from build123d import *
from build123d.topology import SkipClean

# Parameters (mm, degrees)
BOSS_EXTRUDE1_DEPTH     = 12
CUT_EXTRUDE1_DEPTH      = 22.914607001
CUT_EXTRUDE1_DEPTH_BACK = 22.914607001
SKETCH4_R               = 3
SKETCH4_R_2             = 1.5
BOSS_EXTRUDE2_DEPTH     = 8
SKETCH5_R               = 3
SKETCH5_R_2             = 1.5
CUT_EXTRUDE2_DEPTH      = 2.5
FILLET1_R               = 1
FILLET2_R               = 1
CUT_EXTRUDE3_DEPTH      = 22.914607001
CUT_EXTRUDE3_DEPTH_BACK = 22.914607001
SKETCH6_W               = 12
SKETCH6_H               = 6.5
CUT_EXTRUDE4_DEPTH      = 5
BOSS_EXTRUDE3_REACH     = 24.623
SKETCH8_R               = 1.5
SKETCH9_W               = 2
SKETCH9_H               = 33.212886517
CUT_EXTRUDE5_DEPTH      = 1


with BuildPart() as part:
    # Sketch1 → Boss-Extrude1 (new body)
    with BuildSketch(Plane.XY):
        with BuildLine():
            Line((-8, -10), (8, -10))
            Line((8, -10), (6.5, 10))
            ThreePointArc((6.5, 10), (0, 16.5), (-6.5, 10))
            Line((-6.5, 10), (-8, -10))
        make_face()
    extrude(amount=BOSS_EXTRUDE1_DEPTH)

    # Sketch3 → Cut-Extrude1 (cut, two sides: drawn at the far end of the back side and taken through both)
    with BuildSketch(Plane(origin=(0, 0, 0), x_dir=(0, 0, -1), z_dir=(1, 0, 0)).offset(-CUT_EXTRUDE1_DEPTH_BACK)):
        Polygon((-4, -10), (-12, -3.386045056), (-12, -10), align=None)
    extrude(amount=CUT_EXTRUDE1_DEPTH + CUT_EXTRUDE1_DEPTH_BACK, mode=Mode.SUBTRACT)

    # Sketch4 → Boss-Extrude2 (add, symmetric)
    with BuildSketch(Plane(origin=(0, 0, 0), x_dir=(0, 0, -1), z_dir=(1, 0, 0))):
        with Locations((-6, -11.1)):
            Circle(SKETCH4_R)
        with Locations((-6, -11.1)):
            Circle(SKETCH4_R_2, mode=Mode.SUBTRACT)
    extrude(amount=BOSS_EXTRUDE2_DEPTH, both=True)

    # Sketch5 → Cut-Extrude2 (cut, symmetric)
    with SkipClean():  # the faces are left unmerged after this step: merging them gives an invalid solid
        with BuildSketch(Plane(origin=(0, 0, 0), x_dir=(0, 0, -1), z_dir=(1, 0, 0))):
            with Locations((-6, -11.1)):
                Circle(SKETCH5_R)
            with Locations((-6, -11.1)):
                Circle(SKETCH5_R_2, mode=Mode.SUBTRACT)
        extrude(amount=CUT_EXTRUDE2_DEPTH, both=True, mode=Mode.SUBTRACT)

    # Fillet1
    fillet1_edges = [part.edges().sort_by_distance(p)[0] for p in [
        (5.179248458, -8.113292219, 6.282093298),
        (-5.179248458, -8.113292219, 6.282093298),
    ]]
    fillet(fillet1_edges, radius=FILLET1_R)

    # Fillet2
    # the kernel refuses this fillet: 1 mm, written as the material it adds along each edge
    with BuildSketch(Plane(origin=(-8, -10, 3.208942853), x_dir=(0, 0, -1), z_dir=(1, 0, 0)), Plane(origin=(2.5, -10, 3.208942853), x_dir=(0, 0, -1), z_dir=(1, 0, 0))) as fillet2_piece_1:
        with BuildLine():
            CenterArc((1.207692657, -1), FILLET2_R, 90, 91.432543738)
            ThreePointArc((0.208005206, -1.025), (0.149015506, -0.503365446), (0, 0))
            Line((0, 0), (1.207692657, 0))
        make_face()
    extrude(amount=5.5)

    # Sketch6 → Cut-Extrude3 (cut, two sides: drawn at the far end of the back side and taken through both)
    with BuildSketch(Plane(origin=(0, 0, 0), x_dir=(0, 0, -1), z_dir=(1, 0, 0)).offset(-CUT_EXTRUDE3_DEPTH_BACK)):
        with Locations((-6, 13.25)):
            Rectangle(SKETCH6_W, SKETCH6_H)
    extrude(amount=CUT_EXTRUDE3_DEPTH + CUT_EXTRUDE3_DEPTH_BACK, mode=Mode.SUBTRACT)

    # Sketch7 → Cut-Extrude4 (cut)
    with BuildSketch(Plane(origin=(0, -7.904323178, 6.53485467), x_dir=(1, 0, 0), z_dir=(0, -0.770712909441233, 0.6371825572162423))):
        Polygon((-5, 5.891026066), (0, 5.891026066), (5, 5.891026066), (5, 1.891026066), (-5, 1.891026066), align=None)
    extrude(amount=-CUT_EXTRUDE4_DEPTH, mode=Mode.SUBTRACT)

    # Sketch8 → Boss-Extrude3 (add, up to next)
    with BuildSketch(Plane(origin=(-5, 0, 0), x_dir=(0, 0, -1), z_dir=(1, 0, 0)), mode=Mode.PRIVATE) as boss_extrude3_sk1:
        with Locations(Location((-7.940762297, -3.498246966, 0), (0, 0, 180))):
            Circle(SKETCH8_R)
    boss_extrude3_tool1 = extrude(boss_extrude3_sk1.sketch, amount=BOSS_EXTRUDE3_REACH, mode=Mode.PRIVATE) - part.part
    add(boss_extrude3_tool1.solids().sort_by_distance((-5, -3.498247, 7.940762))[0])

    # Sketch9 → Cut-Extrude5 (cut, symmetric)
    with BuildSketch(Plane(origin=(0, 0, 0), x_dir=(0, 0, -1), z_dir=(1, 0, 0))):
        with Locations((-1.32, 6.606443259)):
            Rectangle(SKETCH9_W, SKETCH9_H)
    extrude(amount=CUT_EXTRUDE5_DEPTH, both=True, mode=Mode.SUBTRACT)


solid = part.part
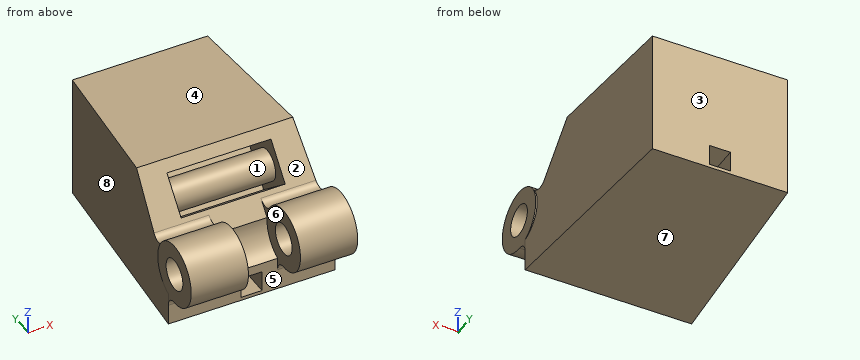
Input: part model. Units: mm. Frame: model coordinates. Face numbers are marked on the shaded views. A direction names the side the tool comes from. Give positions to 0.01 mm unless a question says otherwise; leave off trailing zeros. Order: outer loops, then holes, each group sorted by start corner. A loop starts at its lowest first (then second) coordinate and runs counter-clockwise, first axis right, second up. Notation, with made-up numbers: (65, 54.25) - (119, 54.25) arc R30 cw to (119, 89.25) - close; hole circle Ø5 at (53, -23). An arc over 180 degrees is marked (long way). Answer as a JSON object with one key per item and string values. Group by question number.
Q1. Mould query, pull axis X, two halves, no side actions, for the marked faces 6, 7 and 8. Classes: pulls with the +X half, pulls with the -X half, needs draft (parallel to the pull), parting line crosses it, or undercut.
Q2. Cut plane B-B, the plane z = 8.25. Output: boundary loops of the cut face in (x, y), then the cut area to 3 significant figures.
Q3. Line query: probe 1 along Z at (x, y) = (-3.25, -3); probe 2 along X at (y, z) = (-8.75, 5.5); probe 3 along Y at (x, z) = (6.35, 6). Output: solid intervals per line, ascending.
Q4. Cut plane A-A, the plane x = 4.25. Output: boundary loops of the cut face in (y, z) (3 decimals), then the cut area to 3 significant figures.
Q5. Cut plane C-C, the plane x = -1.75. Output: boundary loops of the cut face in (y, z), then the cut area to 3 significant figures.
Q6. Set-up query: the marked faces 1, 2, 3, 4 and 5. Return all of +Z, -Z, +X, -X, +Y, -Y with unobstructed straight access to the full face (end or side cutting, diameter ignored); none if empty.
Q7. Cut plane D-D, the plane z = 6. Output: boundary loops of the cut face in (x, y).
Q8. First-contact query: pin 1 Ø1.6 at (x, z) = (3.5, 1.5) entering from -Y; pin 2 Ø0.6 at (y, z) = (-0.5, 1.5) entering from -X; pin 3 Ø2 at (y, z) = (-0.5, 1) entering from +X. Flat tips, straight axial feed; report the tip coordinate or a pass-through.
Results:
{
 "1": {"face 6": "undercut", "face 7": "needs draft", "face 8": "pulls with the -X half"},
 "2": {"outline": "(-8, -13.08) - (-2.5, -13.08) - (-2.5, -9.12) - (-8, -9.12) - close; (-7.74, -6.49) - (-5, -6.49) - (-5, -4.97) - (5, -4.97) - (5, -6.49) - (7.74, -6.49) - (6.5, 10) - (-6.5, 10) - close; (2.5, -13.08) - (8, -13.08) - (8, -9.12) - (2.5, -9.12) - close; hole (-5, -2.03) - (5, -2.03) - (5, -0.73) - (-5, -0.73) - close", "area": "250 mm^2"},
 "3": {"probe 1": "0 to 4.93, 6.53 to 9.36, 10.12 to 12", "probe 2": "-8 to -2.5, 2.5 to 8", "probe 3": "-14.1 to -12.6, -9.6 to 10"},
 "4": {"outline": "(-11.025, 3.001) arc R1 cw to (-10, 2.001) - (-10, 0) - (10, 0) - (10, 12) - (-3.386, 12) - (-4.151, 11.075) - (-0.297, 7.889) - (-2.846, 4.806) - (-6.699, 7.992) - (-7.018, 7.607) arc R1 cw to (-8.617, 7.683) arc R3 ccw (long way) to start; circle Ø3 at (-3.498, 7.941); hole circle Ø3 at (-11.1, 6)", "area": "220 mm^2"},
 "5": {"outline": "(-10, 0) - (10, 0) - (10, 12) - (-3.39, 12) - (-4.15, 11.08) - (-0.3, 7.89) - (-2.85, 4.81) - (-6.7, 7.99) - (-8.11, 6.28) arc R3 cw to (-10, 3.21) - close; circle Ø3 at (-3.5, 7.94)", "area": "198 mm^2"},
 "6": {"face 1": "none", "face 2": "+Z", "face 3": "+Z, -Z, +X, -X, +Y", "face 4": "+Z, +X, -X, +Y, -Y", "face 5": "-Z, -Y"},
 "7": {"outline": "(-8, -14.1) - (-2.5, -14.1) - (-2.5, -12.6) - (-8, -12.6) - close; (-8, -9.6) - (-2.5, -9.6) - (-2.5, -8.1) - (2.5, -8.1) - (2.5, -9.6) - (8, -9.6) - (8, -8.1) - (7.86, -8.1) - (6.5, 10) - (-6.5, 10) - (-7.86, -8.1) - (-8, -8.1) - close; (2.5, -14.1) - (8, -14.1) - (8, -12.6) - (2.5, -12.6) - close; hole (-5, -4.29) - (5, -4.29) - (5, -1.86) - (-5, -1.86) - close"},
 "8": {"pin 1": "y = -10.05", "pin 2": "x = -7.31", "pin 3": "x = 7.36"}
}
